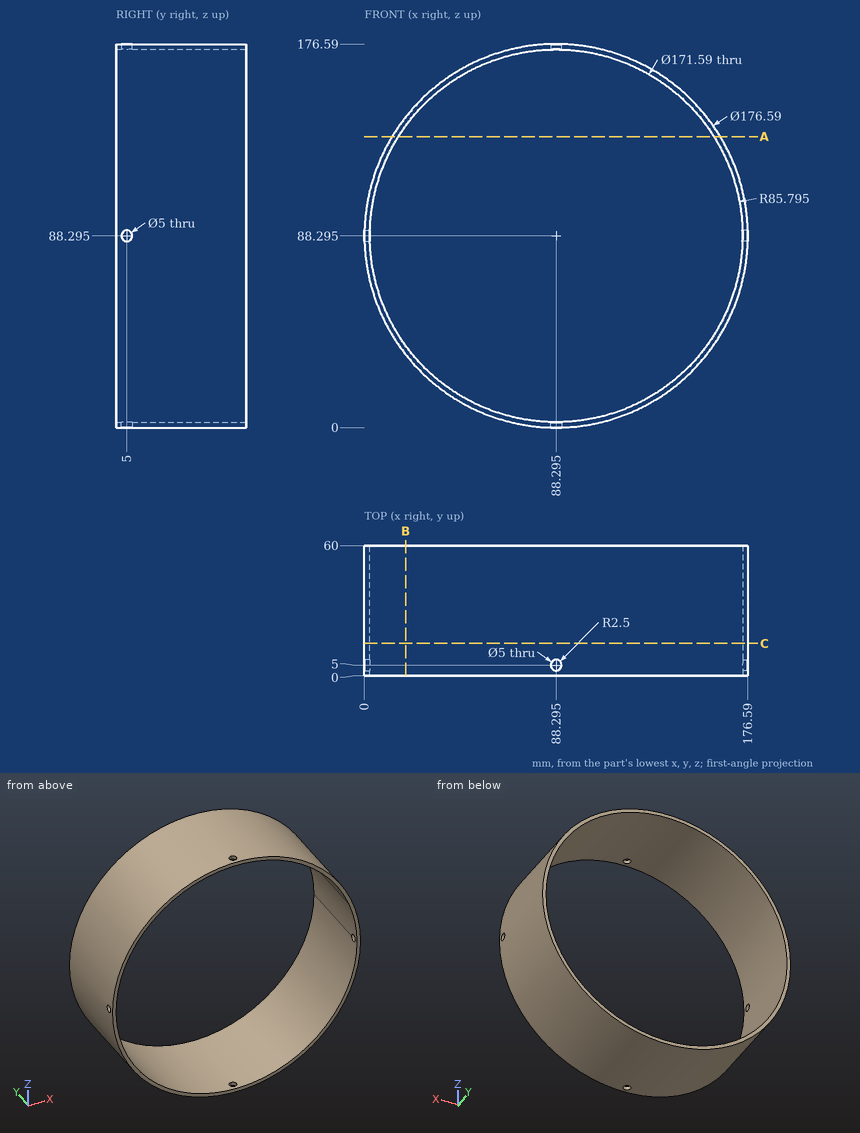
Can you work these out from the drawing? Everything is in mm from the part's minimum corner. Give positions to 0.01 mm unless a question says otherwise; leave off trailing zeros. Loops run counter-clockwise (first coordinate to the right, second up) from the corner with the lowest first, then second, coordinate; pieces in that order, holes last. Notation, with made-up numbers: (79.25, -7) -> (87.25, -7) arc R9 cw to (87.25, 6) -> close; hole circle Ø9 at (78.5, 19). An arc over 180 degrees is marked (long way). Return JSON: item names as keys, results as strings.
Item 1: If we section it at B-B on x = 19: List the corners of the cut face in (y, z) for me.
Geometry results:
{"outline": "(0, 33.58) -> (60, 33.58) -> (60, 37.71) -> (0, 37.71) -> close; (0, 138.88) -> (60, 138.88) -> (60, 143.01) -> (0, 143.01) -> close"}
Item 2: I need wall thicknesses on L1, parallel to X at y = 12.5, z = 88.5; L2, parallel to Z at x = 116.5, y = 47.5; L3, parallel to Z at x = 69, y = 21.5. Which ranges of each line are inside material? Lowest first, please. Write a range as from..to.
Geometry results:
{"L1": "x = 0..2.5, 174.09..176.59", "L2": "z = 4.63..7.27, 169.32..171.96", "L3": "z = 2.13..4.7, 171.89..174.46"}
Item 3: If we section it at C-C on y = 15: List the corners of the cut face in (x, z) for me (3 decimals), plus the area to 3 significant figures.
Geometry results:
{"outline": "circle Ø176.59 at (88.295, 88.295); hole circle Ø171.59 at (88.295, 88.295)", "area": "1,370 mm²"}
Item 4: If we section it at A-A on z = 134: List the corners of the cut face in (x, y) for me, plus the area to 3 significant figures.
Geometry results:
{"outline": "(12.75, 0) -> (15.69, 0) -> (15.69, 60) -> (12.75, 60) -> close; (160.9, 0) -> (163.84, 0) -> (163.84, 60) -> (160.9, 60) -> close", "area": "353 mm²"}
Item 5: I'm going to push flat-ended pins straight in: pin 1 (1 mm diameter, centred on y = 8.5, z = 51.5, fed in from +X); pin 2 (4 mm diameter, centred on x = 72, y = 29, fed in from +Z); pin 3 (8 mm diameter, centred on y = 5, z = 88.295, fed in from +X); pin 4 (3 mm diameter, centred on x = 120, y = 9.5, fed in from -Z). Where does each tip first touch, or does it pass through?
Geometry results:
{"pin 1": "stops at x = 168.79", "pin 2": "stops at z = 175.43", "pin 3": "stops at x = 176.59", "pin 4": "stops at z = 5.33"}
